Autodesk Inventor part; units mm, degrees
ref_plane "YZ Plane" through (0, 0, 0) normal (1, 0, 0) x (0, 1, 0)
ref_plane "XZ Plane" through (0, 0, 0) normal (0, 1, 0) x (-1, 0, 0)
ref_plane "XY Plane" through (0, 0, 0) normal (0, 0, 1) x (1, 0, 0)
sketch "Sketch1" plane through (0, 0, 0) normal (0, 1, 0) x (-1, 0, 0)
  line L0 (17.9605, 0) -> (0, -17.9605)
  line L1 (17.9605, 0) -> (43.3605, 0) construction
  line L2 (17.9605, 0) -> (0, 17.9605)
  line L3 (17.9605, 0) -> (43.3605, 0) construction
  line L4 (-17.9605, 0) -> (0, -17.9605)
  line L5 (-17.9605, 0) -> (0, 17.9605)
  line L6 (0, 15.4205) -> (-15.4205, 0)
  line L7 (0, 15.4205) -> (21.8079, 15.4205) construction
  line L8 (-15.4205, 0) -> (0, -15.4205)
  line L9 (0, -15.4205) -> (15.4205, 0)
  line L10 (15.4205, 0) -> (0, 15.4205)
  line L11 (0, -40.8205) -> (2, -40.8205)
  line L12 (0, -40.8205) -> (-2, -40.8205)
  circle A0 centre (7.5, -28.1205) radius 2.5
  line L13 (4, -28.1205) -> (4, -13.9605)
  line L14 (4, -28.1205) -> (4, -40.8205)
  line L15 (11, -6.9605) -> (11, -40.8205)
  arc A1 (-4, -40.8205) -> (4, -40.8205) centre (0, -40.8205) ccw
  line L16 (0, -15.4205) -> (0, -17.9605)
  line L17 (-4, -40.8205) -> (-4, -13.9605)
  line L18 (-11, -40.8205) -> (-11, -6.9605)
  arc A2 (-11, -40.8205) -> (11, -40.8205) centre (0, -40.8205) ccw
  circle A3 centre (-7.5, -24.8705) radius 2.5
  circle A4 centre (-7.5, -36.6205) radius 2.5
  line L19 (15.4205, 0) -> (17.9605, 0)
  line L20 (28.1205, 4) -> (13.9605, 4)
  circle A5 centre (28.1205, 7.5) radius 2.5
  circle A6 centre (24.8705, -7.5) radius 2.5
  line L21 (6.9605, 11) -> (40.8205, 11)
  line L22 (40.8205, -11) -> (6.9605, -11)
  line L23 (40.8205, -4) -> (13.9605, -4)
  line L24 (28.1205, 4) -> (40.8205, 4)
  line L25 (40.8205, 0) -> (40.8205, 2)
  circle A7 centre (36.6205, -7.5) radius 2.5
  line L26 (40.8205, 0) -> (40.8205, -2)
  arc A8 (40.8205, -4) -> (40.8205, 4) centre (40.8205, 0) ccw
  arc A9 (40.8205, -11) -> (40.8205, 11) centre (40.8205, 0) ccw
  line L27 (0, 15.4205) -> (0, 17.9605)
  line L28 (-4, 28.1205) -> (-4, 13.9605)
  circle A10 centre (-7.5, 28.1205) radius 2.5
  circle A11 centre (7.5, 24.8705) radius 2.5
  line L29 (-11, 6.9605) -> (-11, 40.8205)
  line L30 (11, 40.8205) -> (11, 6.9605)
  line L31 (4, 40.8205) -> (4, 13.9605)
  line L32 (-4, 28.1205) -> (-4, 40.8205)
  line L33 (0, 40.8205) -> (-2, 40.8205)
  circle A12 centre (7.5, 36.6205) radius 2.5
  line L34 (0, 40.8205) -> (2, 40.8205)
  arc A13 (4, 40.8205) -> (-4, 40.8205) centre (0, 40.8205) ccw
  arc A14 (11, 40.8205) -> (-11, 40.8205) centre (0, 40.8205) ccw
  line L35 (-15.4205, 0) -> (-17.9605, 0)
  line L36 (-28.1205, -4) -> (-13.9605, -4)
  circle A15 centre (-28.1205, -7.5) radius 2.5
  circle A16 centre (-24.8705, 7.5) radius 2.5
  line L37 (-6.9605, -11) -> (-40.8205, -11)
  line L38 (-40.8205, 11) -> (-6.9605, 11)
  line L39 (-40.8205, 4) -> (-13.9605, 4)
  line L40 (-28.1205, -4) -> (-40.8205, -4)
  line L41 (-40.8205, 0) -> (-40.8205, -2)
  circle A17 centre (-36.6205, 7.5) radius 2.5
  line L42 (-40.8205, 0) -> (-40.8205, 2)
  arc A18 (-40.8205, 4) -> (-40.8205, -4) centre (-40.8205, 0) ccw
  arc A19 (-40.8205, 11) -> (-40.8205, -11) centre (-40.8205, 0) ccw
  point P0 (0, 0)
  point P1 (0, -28.1205)
  point P2 (2, -28.1205)
  point P3 (-2, -22.1205)
  point P4 (-7.5, -22.1205)
  point P5 (-2, -34.1205)
  point P6 (-7.5, -34.1205)
  point P7 (11, -28.1205)
  point P8 (28.1205, 2)
  point P9 (28.1205, 11)
  point P10 (34.1205, -7.5)
  point P11 (34.1205, -2)
  point P12 (22.1205, -7.5)
  point P13 (22.1205, -2)
  point P14 (28.1205, 0)
  point P15 (-2, 28.1205)
  point P16 (-11, 28.1205)
  point P17 (7.5, 34.1205)
  point P18 (2, 34.1205)
  point P19 (7.5, 22.1205)
  point P20 (2, 22.1205)
  point P21 (0, 28.1205)
  point P22 (-28.1205, -2)
  point P23 (-28.1205, -11)
  point P24 (-34.1205, 7.5)
  point P25 (-34.1205, 2)
  point P26 (-22.1205, 7.5)
  point P27 (-22.1205, 2)
  point P28 (-28.1205, 0)
  point P29 (11, 11)
  point P30 (-11, 11)
  point P31 (-11, -11)
  point P32 (11, -11)
  dimension "d12" = 25.4
  dimension "d15" = 25.4
  dimension "d18" = 2.54
  dimension "d19" = 135
  dimension "d25" = 5
  dimension "d41" = 360
extrude "Extrusion1" add sketch "Sketch1" along normal blind 6 contours L19 L10 L27 L2 | L0 L16 L9 L19 | L23 A8 L24 L20 L2 L30 L21 A9 L22 L15 L0 | L9 L8 L6 L10 | L15 L22 L0 | L2 L21 L30 | L16 L4 L35 L8 | L6 L35 L5 L27 | L22 L15 A2 L18 L37 L4 L17 A1 L14 L13 L0 | L2 L31 A13 L32 L28 L5 L38 L29 A14 L30 L21 | L4 L18 L37 A19 L38 L29 L5 L39 A18 L40 L36 | L37 L18 L4 | L5 L29 L38 | A0 | A3 | A4 | A5 | A6 | A7 | A10 | A11 | A12 | A15 | A16 | A17
extrude "Extrusion2" add sketch "Sketch1" against normal blind 5.6 contours A0 | A3 | A4 | A5 | A6 | A7 | A10 | A11 | A12 | A15 | A16 | A17
sketch "Sketch2" plane through (0, 0, 0) normal (0, -1, 0) x (1, 0, 0)
  circle A0 centre (7.5, 28.1205) radius 2.5
  circle A1 centre (7.5, 28.1205) radius 2.625
  circle A2 centre (-7.5, 36.6205) radius 2.5
  circle A3 centre (-7.5, 36.6205) radius 2.625
  circle A4 centre (-7.5, 24.8705) radius 2.5
  circle A5 centre (-7.5, 24.8705) radius 2.625
  circle A6 centre (-28.1205, 7.5) radius 2.625
  circle A7 centre (-36.6205, -7.5) radius 2.625
  circle A8 centre (-24.8705, -7.5) radius 2.625
  circle A9 centre (-7.5, -28.1205) radius 2.625
  circle A10 centre (7.5, -36.6205) radius 2.625
  circle A11 centre (7.5, -24.8705) radius 2.625
  circle A12 centre (28.1205, -7.5) radius 2.625
  circle A13 centre (36.6205, 7.5) radius 2.625
  circle A14 centre (24.8705, 7.5) radius 2.625
  point P0 (0, 0)
  dimension "d47" = 5.25
  dimension "d48" = 5.25
  dimension "d49" = 5.25
  dimension "d52" = 360
extrude "Extrusion3" add sketch "Sketch2" along normal blind 0.6 contours A0 | A1 | A2 | A3 | A4 | A5 | A6 | A7 | A8 | A9 | A10 | A11 | A12 | A13 | A14
sketch "Sketch3" plane through (7.5, -5.6, 28.1205) normal (0, -1, 0) x (1, 0, 0)
  circle A0 centre (0, 0) radius 2
  circle A1 centre (-15, 8.5) radius 2.5
  circle A2 centre (-15, 8.5) radius 2
  circle A3 centre (-15, -3.25) radius 2.5
  circle A4 centre (-15, -3.25) radius 2
  circle A5 centre (-44.1205, -35.6205) radius 2
  circle A6 centre (-32.3705, -35.6205) radius 2
  circle A7 centre (-35.6205, -20.6205) radius 2
  circle A8 centre (0, -64.741) radius 2
  circle A9 centre (0, -52.991) radius 2
  circle A10 centre (-15, -56.241) radius 2
  circle A11 centre (29.1205, -20.6205) radius 2
  circle A12 centre (17.3705, -20.6205) radius 2
  circle A13 centre (20.6205, -35.6205) radius 2
  point P0 (-7.5, -28.1205)
  dimension "d56" = 4
  dimension "d57" = 4
  dimension "d58" = 4
  dimension "d61" = 360
extrude "Extrusion4" cut sketch "Sketch3" against normal blind 6 contours A0 | A2 | A4 | A5 | A6 | A7 | A8 | A9 | A10 | A11 | A12 | A13
properties part number "Redesign_Gripper_Baseplate"
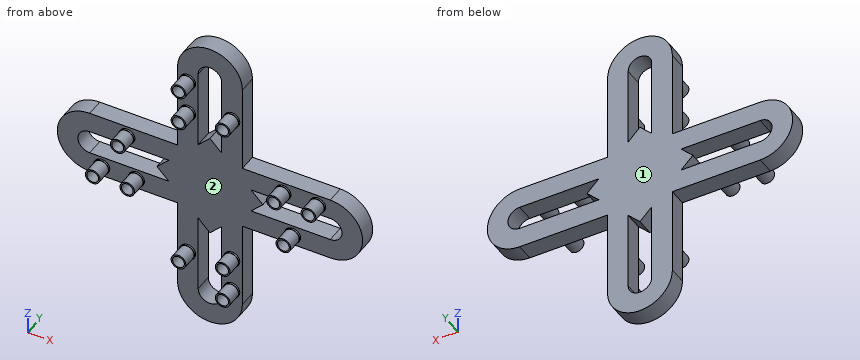
Build history of the part. All positions in model axes, mm. Face numbers are marked on the shaded views. Coordinates: 2 decimals unless noted, no trailing zeros. Use CSV: the item, a comma, the result in double quotes. Start each with the question number.
Q1. Pull direction X, two halves, no side cores. Call the marked faces 1 and 2: released by +X, released by -X, zero draft, split by the parting line, or undercut.
Q2. Cut at A-A, the plane y = -3.5. State how many separate pieces and enclosed holes the cut face has, then the cut area to 3 significant figures.
Q3. Drill centre lines: probe 1 along Z at (x, y) = (-7.5, -1.4); probe 2 along Z at (x, y) = (0, 3); probe 3 along Z at (x, y) = (7.5, -3.4). Where is each one in solid material? Low to high.
Q4. Flat gauge pins, fed straight in: pin 1 Ø2 at (x, y) = (7.5, 2.5) entering from +Z; pin 2 Ø1 at (y, z) = (0.5, -20) entering from -X; pin 3 Ø3 at (x, y) = (-22, 3.5) entering from +Z. Where does each tip first touch, or does it go through?
Checked values:
1,face 1,"zero draft"
1,face 2,"undercut"
2,separate pieces,"12"
2,enclosed holes,"12"
2,area,"84.8 mm²"
3,probe 1,"z = -30.62 to -30.12, -26.12 to -25.62, 22.37 to 22.87, 26.87 to 27.37, 34.12 to 34.62, 38.62 to 39.12"
3,probe 2,"z = -51.82 to -44.82, -17.96 to 17.96, 44.82 to 51.82"
3,probe 3,"z = -39.12 to -38.62, -34.62 to -34.12, -27.37 to -26.87, -22.87 to -22.37, 25.62 to 26.12, 30.12 to 30.62"
4,pin 1,"stops at z = 49.69"
4,pin 2,"stops at x = -11"
4,pin 3,"stops at z = 11"
